Part model, mm, in its own coordinate system. A direction names the side the tool comes from. Round coordinates to 2 decimals unless told otherwise and drop trailing zeros.
1) Flat gauge pins, fed straight in: pin 1 (1 mm diameter, centred on y = 19.5, z = -11, fed in from +X); pin 2 (1 mm diameter, centred on x = 6, y = 9, fed in from +Z); pin 3 (1.3 mm diameter, centred on x = -2.5, z = -13.5, fed in from -Y). Where does each tip first touch, or does it go through?
2) Pull direction Z, two halves, no side cores. Call faces 1 (the flat face through (13.4, 20, 2.2)), 2 (the flat face through (-1, 9.9, 13.6)): +Z half, -Z half, draft (parallel to the pull), parting line (faces both ways), or undercut.
3) Drill centre lines: L1, parallel to X at y = 21.05, z = 0; L2, parallel to Z at x = 0, y = 13.25; L3, parallel to Z at x = 0, y = 23.05. Where is each one in solid material? Low to high.
4) Which spindle directions (+Z, -Z, +X, -X, +Y, -Y) get a long thin tool onto all of the face, cutting with end or side? Do faces 3 (the cylindrical face through (-10.978, 20.74, -2.438)), 4 (the flat face through (-4, 0, -13)), 5 (the cylindrical face through (-9.36, 10.11, -9.38)), 6 (the cylindrical face through (13.09, 10.11, -2.06)). Say none if no direction does.
```python
from build123d import *
from build123d.topology import SkipClean

# Parameters (mm, degrees)
SKETCH_1_R      = 13.25
EXTRUDE_1_DEPTH = 25
SHELL_1_T       = -2
CHAMFER_1_SIZE  = 0.5
EXTRUDE_2_DEPTH = 20
SKETCH_3_R      = 14.05
SKETCH_3_R_2    = 11.244970287
EXTRUDE_3_DEPTH = 1.5


with BuildPart() as part:
    # 草图1 → 拉伸1 (new body)
    with BuildSketch(Plane(origin=(0, 0, 0), x_dir=(1, 0, 0), z_dir=(0, 1, 0))):
        with Locations(Location((0, 0, 0), (0, 0, 270))):
            Circle(SKETCH_1_R)
    extrude(amount=EXTRUDE_1_DEPTH)

    # 抽壳1
    shell_1_openings = [part.faces().sort_by_distance(p)[0] for p in [
        (0, 25, 0),
    ]]
    offset(amount=SHELL_1_T, openings=shell_1_openings, kind=Kind.INTERSECTION)

    # 倒角1
    chamfer_1_edges = [part.edges().sort_by_distance(p)[0] for p in [
        (0, 0, -13.25),
    ]]
    chamfer(chamfer_1_edges, length=CHAMFER_1_SIZE)

    # 草图2 → 拉伸2 (add)
    with BuildSketch(Plane.XZ):
        with BuildLine():
            Line((5.03385402, 12.25654167), (5.281734279, 13.01943866))
            ThreePointArc((5.281734279, 13.01943866), (4.341688771, 13.362344054), (3.379621246, 13.637472648))
            Line((3.379621246, 13.637472648), (3.131740988, 12.874575658))
            ThreePointArc((3.131740988, 12.874575658), (4.094475175, 12.601498841), (5.03385402, 12.25654167))
        make_face()
        with BuildLine():
            Line((1, 13.212210262), (1, 14.014367628))
            ThreePointArc((1, 14.014367628), (0, 14.05), (-1, 14.014367628))
            Line((-1, 14.014367628), (-1, 13.212210262))
            ThreePointArc((-1, 13.212210262), (0, 13.25), (1, 13.212210262))
        make_face()
        with BuildLine():
            Line((8.574959336, 10.101117383), (9.046455606, 10.750076324))
            ThreePointArc((9.046455606, 10.750076324), (8.258382795, 11.366688771), (7.428421617, 11.925646828))
            Line((7.428421617, 11.925646828), (6.956925348, 11.276687887))
            ThreePointArc((6.956925348, 11.276687887), (7.788154593, 10.719475175), (8.574959336, 10.101117383))
        make_face()
        with BuildLine():
            Line((11.276687887, 6.956925348), (11.925646828, 7.428421617))
            ThreePointArc((11.925646828, 7.428421617), (11.366688771, 8.258382795), (10.750076324, 9.046455606))
            Line((10.750076324, 9.046455606), (10.101117383, 8.574959336))
            ThreePointArc((10.101117383, 8.574959336), (10.719475175, 7.788154593), (11.276687887, 6.956925348))
        make_face()
        with BuildLine():
            Line((12.874575658, 3.131740988), (13.637472648, 3.379621246))
            ThreePointArc((13.637472648, 3.379621246), (13.362344054, 4.341688771), (13.01943866, 5.281734279))
            Line((13.01943866, 5.281734279), (12.25654167, 5.03385402))
            ThreePointArc((12.25654167, 5.03385402), (12.601498841, 4.094475175), (12.874575658, 3.131740988))
        make_face()
        with BuildLine():
            Line((13.212210262, -1), (14.014367628, -1))
            ThreePointArc((14.014367628, -1), (14.05, 0), (14.014367628, 1))
            Line((14.014367628, 1), (13.212210262, 1))
            ThreePointArc((13.212210262, 1), (13.25, 0), (13.212210262, -1))
        make_face()
        with BuildLine():
            Line((12.25654167, -5.03385402), (13.01943866, -5.281734279))
            ThreePointArc((13.01943866, -5.281734279), (13.362344054, -4.341688771), (13.637472648, -3.379621246))
            Line((13.637472648, -3.379621246), (12.874575658, -3.131740988))
            ThreePointArc((12.874575658, -3.131740988), (12.601498841, -4.094475175), (12.25654167, -5.03385402))
        make_face()
        with BuildLine():
            Line((10.101117383, -8.574959336), (10.750076324, -9.046455606))
            ThreePointArc((10.750076324, -9.046455606), (11.366688771, -8.258382795), (11.925646828, -7.428421617))
            Line((11.925646828, -7.428421617), (11.276687887, -6.956925348))
            ThreePointArc((11.276687887, -6.956925348), (10.719475175, -7.788154593), (10.101117383, -8.574959336))
        make_face()
        with BuildLine():
            Line((6.956925348, -11.276687887), (7.428421617, -11.925646828))
            ThreePointArc((7.428421617, -11.925646828), (8.258382795, -11.366688771), (9.046455606, -10.750076324))
            Line((9.046455606, -10.750076324), (8.574959336, -10.101117383))
            ThreePointArc((8.574959336, -10.101117383), (7.788154593, -10.719475175), (6.956925348, -11.276687887))
        make_face()
        with BuildLine():
            Line((3.131740988, -12.874575658), (3.379621246, -13.637472648))
            ThreePointArc((3.379621246, -13.637472648), (4.341688771, -13.362344054), (5.281734279, -13.01943866))
            Line((5.281734279, -13.01943866), (5.03385402, -12.25654167))
            ThreePointArc((5.03385402, -12.25654167), (4.094475175, -12.601498841), (3.131740988, -12.874575658))
        make_face()
        with BuildLine():
            Line((-1, -13.212210262), (-1, -14.014367628))
            ThreePointArc((-1, -14.014367628), (0, -14.05), (1, -14.014367628))
            Line((1, -14.014367628), (1, -13.212210262))
            ThreePointArc((1, -13.212210262), (0, -13.25), (-1, -13.212210262))
        make_face()
        with BuildLine():
            Line((-5.03385402, -12.25654167), (-5.281734279, -13.01943866))
            ThreePointArc((-5.281734279, -13.01943866), (-4.341688771, -13.362344054), (-3.379621246, -13.637472648))
            Line((-3.379621246, -13.637472648), (-3.131740988, -12.874575658))
            ThreePointArc((-3.131740988, -12.874575658), (-4.094475175, -12.601498841), (-5.03385402, -12.25654167))
        make_face()
        with BuildLine():
            Line((-8.574959336, -10.101117383), (-9.046455606, -10.750076324))
            ThreePointArc((-9.046455606, -10.750076324), (-8.258382795, -11.366688771), (-7.428421617, -11.925646828))
            Line((-7.428421617, -11.925646828), (-6.956925348, -11.276687887))
            ThreePointArc((-6.956925348, -11.276687887), (-7.788154593, -10.719475175), (-8.574959336, -10.101117383))
        make_face()
        with BuildLine():
            Line((-11.276687887, -6.956925348), (-11.925646828, -7.428421617))
            ThreePointArc((-11.925646828, -7.428421617), (-11.366688771, -8.258382795), (-10.750076324, -9.046455606))
            Line((-10.750076324, -9.046455606), (-10.101117383, -8.574959336))
            ThreePointArc((-10.101117383, -8.574959336), (-10.719475175, -7.788154593), (-11.276687887, -6.956925348))
        make_face()
        with BuildLine():
            Line((-12.874575658, -3.131740988), (-13.637472648, -3.379621246))
            ThreePointArc((-13.637472648, -3.379621246), (-13.362344054, -4.341688771), (-13.01943866, -5.281734279))
            Line((-13.01943866, -5.281734279), (-12.25654167, -5.03385402))
            ThreePointArc((-12.25654167, -5.03385402), (-12.601498841, -4.094475175), (-12.874575658, -3.131740988))
        make_face()
        with BuildLine():
            Line((-13.212210262, 1), (-14.014367628, 1))
            ThreePointArc((-14.014367628, 1), (-14.05, 0), (-14.014367628, -1))
            Line((-14.014367628, -1), (-13.212210262, -1))
            ThreePointArc((-13.212210262, -1), (-13.25, 0), (-13.212210262, 1))
        make_face()
        with BuildLine():
            Line((-12.25654167, 5.03385402), (-13.01943866, 5.281734279))
            ThreePointArc((-13.01943866, 5.281734279), (-13.362344054, 4.341688771), (-13.637472648, 3.379621246))
            Line((-13.637472648, 3.379621246), (-12.874575658, 3.131740988))
            ThreePointArc((-12.874575658, 3.131740988), (-12.601498841, 4.094475175), (-12.25654167, 5.03385402))
        make_face()
        with BuildLine():
            Line((-10.101117383, 8.574959336), (-10.750076324, 9.046455606))
            ThreePointArc((-10.750076324, 9.046455606), (-11.366688771, 8.258382795), (-11.925646828, 7.428421617))
            Line((-11.925646828, 7.428421617), (-11.276687887, 6.956925348))
            ThreePointArc((-11.276687887, 6.956925348), (-10.719475175, 7.788154593), (-10.101117383, 8.574959336))
        make_face()
        with BuildLine():
            Line((-6.956925348, 11.276687887), (-7.428421617, 11.925646828))
            ThreePointArc((-7.428421617, 11.925646828), (-8.258382795, 11.366688771), (-9.046455606, 10.750076324))
            Line((-9.046455606, 10.750076324), (-8.574959336, 10.101117383))
            ThreePointArc((-8.574959336, 10.101117383), (-7.788154593, 10.719475175), (-6.956925348, 11.276687887))
        make_face()
        with BuildLine():
            Line((-3.131740988, 12.874575658), (-3.379621246, 13.637472648))
            ThreePointArc((-3.379621246, 13.637472648), (-4.341688771, 13.362344054), (-5.281734279, 13.01943866))
            Line((-5.281734279, 13.01943866), (-5.03385402, 12.25654167))
            ThreePointArc((-5.03385402, 12.25654167), (-4.094475175, 12.601498841), (-3.131740988, 12.874575658))
        make_face()
    extrude(amount=-EXTRUDE_2_DEPTH)

    # 草图3 → 拉伸3 (add)
    with SkipClean():  # the faces are left unmerged after this step: merging them gives an invalid solid
        with BuildSketch(Plane(origin=(0, 20, 0), x_dir=(1, 0, 0), z_dir=(0, 1, 0))):
            with Locations(Location((0, 0, 0), (0, 0, 85.91855766))):
                Circle(SKETCH_3_R)
            with Locations(Location((0, 0, 0), (0, 0, 270))):
                Circle(SKETCH_3_R_2, mode=Mode.SUBTRACT)
        extrude(amount=EXTRUDE_3_DEPTH)


solid = part.part
```
Completed:
1. pin 1: stops at x = 9.05
1. pin 2: stops at z = 12.05
1. pin 3: stops at y = 0.33
2. face 1: undercut
2. face 2: draft
3. L1: x = -14.05 to -11.24, 11.24 to 14.05
3. L2: z = -14.05 to -11.25, 11.25 to 14.05
3. L3: z = -13.25 to -11.25, 11.25 to 13.25
4. face 3: +Y
4. face 4: +Z, -Z, +X, -X, -Y
4. face 5: -Y
4. face 6: +X, -Y
